The listing builds one solid part. Answer for the finished solid, in the listing's coordinates (mm). Face numbers are marked on the shaded views. A direction names the side the tool comes from. Round coordinates to 2 decimals unless told otherwise and drop trailing zeros. Loops run counter-clockwise (first coordinate to the right, second up) from the corner with the lowest first, then second, coordinate; pieces in that order, holes last. Notation, with made-up numbers: (88.25, 15.25) -> (105.25, 15.25) arc R21 ccw to (105.25, 29.25) -> close; hole circle Ø2 at (79.25, 18.5). An arc over 180 degrees is marked (long way). Write each question's results on one line, items separated by ' | '. Start each with the question number.
(1) Straight lines are drawn through the part: probe 1 along X at (y, z) = (-146.05, 0.5); probe 2 along Z at (x, y) = (13, -87); probe 3 along Z at (x, y) = (13.25, -138). For each, find the intervals that lie inside material, in ascending order.
(2) For the marked faces 1 and 2, determine the directions among +Z, -Z, +X, -X, +Y, -Y from which every point of the face is accessible in a straight line to the end or side of a thin tool.
(3) The part is cut by section A-A (y = -186). Determine the outline of the cut face in (x, z) (1 decimal).
(4) Flat-ended cylindrical pins translate along their axes: pin 1 (3.5 mm diameter, centred on x = 5.08, y = -69.85, fed in from -Z); pin 2 (5 mm diameter, centred on x = 8, y = -205.5, fed in from +Z); pin 3 (1.2 mm diameter, centred on y = -95, z = 0.5, fed in from +X). Find the tip coordinate at first contact, or state that the pin passes through.
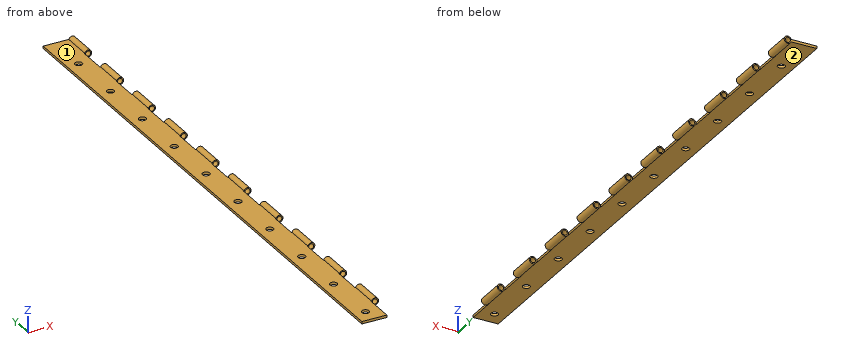
```python
from build123d import *

# Parameters (mm, degrees)
F0_R     = 1.11125
F1_DEPTH = 254
F2_W     = 3.7465
F2_H     = 12.7
F3_DEPTH = 12.7
F4_R     = 1.5875
F5_DEPTH = 25.4


with BuildPart() as f1:
    # F0 (on Front) → F1 (new body)
    with BuildSketch(Plane.XZ):
        with BuildLine():
            Line((0, 1.0668), (0, 0))
            Line((0, 0), (11.204794, 0))
            ThreePointArc((11.204794, 0), (14.2875, 0.5334), (11.204794, 1.0668))
            Line((11.204794, 1.0668), (0, 1.0668))
        make_face()
        with Locations((12.7, 0.5334)):
            Circle(F0_R, mode=Mode.SUBTRACT)
    extrude(amount=F1_DEPTH)

    # F2 (on face) → F3 (cut, symmetric)
    with BuildSketch(Plane.XY.offset(1.0668)):
        with Locations((12.824044, -247.65)):
            Rectangle(F2_W, F2_H)
        with Locations((12.824044, -222.25)):
            Rectangle(F2_W, F2_H)
        with Locations((12.824044, -196.85)):
            Rectangle(F2_W, F2_H)
        with Locations((12.824044, -171.45)):
            Rectangle(F2_W, F2_H)
        with Locations((12.824044, -146.05)):
            Rectangle(F2_W, F2_H)
        with Locations((12.824044, -120.65)):
            Rectangle(F2_W, F2_H)
        with Locations((12.824044, -95.25)):
            Rectangle(F2_W, F2_H)
        with Locations((12.824044, -69.85)):
            Rectangle(F2_W, F2_H)
        with Locations((12.824044, -44.45)):
            Rectangle(F2_W, F2_H)
        with Locations((12.824044, -19.05)):
            Rectangle(F2_W, F2_H)
    extrude(amount=F3_DEPTH, both=True, mode=Mode.SUBTRACT)

    # F4 (on face) → F5 (cut)
    with BuildSketch(Plane.XY.offset(1.0668)):
        with Locations((5.08, -247.65)):
            Circle(F4_R)
        with Locations((5.08, -222.25)):
            Circle(F4_R)
        with Locations((5.08, -196.85)):
            Circle(F4_R)
        with Locations((5.08, -171.45)):
            Circle(F4_R)
        with Locations((5.08, -146.05)):
            Circle(F4_R)
        with Locations((5.08, -120.65)):
            Circle(F4_R)
        with Locations((5.08, -95.25)):
            Circle(F4_R)
        with Locations((5.08, -69.85)):
            Circle(F4_R)
        with Locations((5.08, -44.45)):
            Circle(F4_R)
        with Locations((5.08, -19.05)):
            Circle(F4_R)
    extrude(amount=-F5_DEPTH, mode=Mode.SUBTRACT)


solid = f1.part
```
Checked values:
1) probe 1: x = 0 to 3.49, 6.67 to 10.95 | probe 2: z = -1.03 to -0.54, 1.6 to 2.09 | probe 3: z = -0.96 to -0.43, 1.5 to 2.02
2) face 1: +Z, -X, +Y, -Y | face 2: -Z, -X, +Y, -Y
3) outline: (0, 0) -> (11.2, 0) arc R1.6 ccw (long way) to (11.2, 1.1) -> (0, 1.1) -> close; hole circle Ø2.2 at (12.7, 0.5)
4) pin 1: stops at z = 0 | pin 2: stops at z = 1.07 | pin 3: stops at x = 10.95
